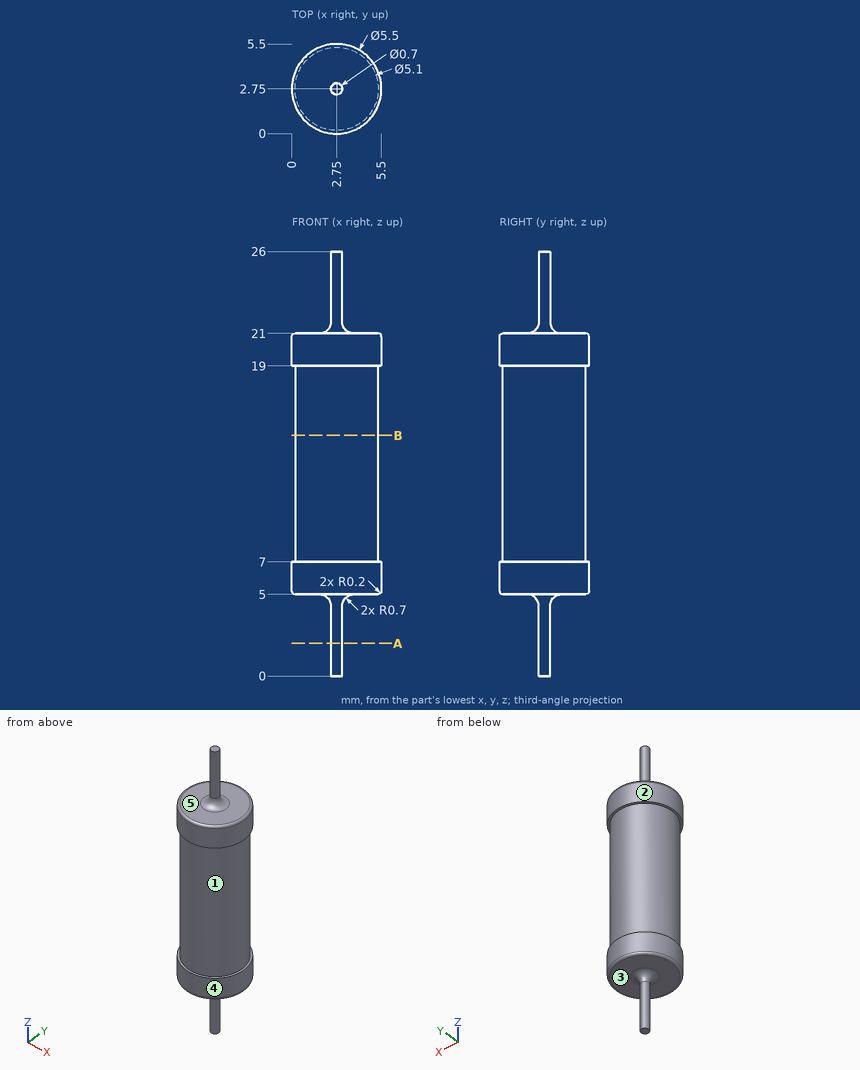
Design review of the part shown in the three views and the two pictorial views. Dimensions are in mm from the part's minimum x, y and z. A direction names the side the tool comes from. Coordinates: 2 decimals unless noted, no trailing zeros. Order: outer loops, then holes, each group sorted by start corner. A loop starts at its lowest first (then second) coordinate and runs counter-clockwise, first axis right, second up.
Item 1: For line 1 (Z direction, x = 4.5, y = 1.5); line 2 (Y direction, x = 2.75, z = 15); line 3 (Y direction, x = 0.45, z = 17), list the stretches that pass through material, from the lowest coordinate up.
Item 2: The part is to be moulded in two halves that separate along Z. For the marked faces 1, 2 and 3, say which applies: pulls with the +Z half, pulls with the -Z half, needs draft (parallel to the pull), parting line crosses it, or undercut.
Item 3: For the marked faces 4 and 5, list the 3-axis set-ups (+Z, -Z, +X, -X, +Y, -Y) from which the entire face can be reached by the end or side of a thin tool; tool diameter is ignored.
Item 4: Take a section at A-A, the plane z = 2. Write out the cut boundary in (x, y), then the cut area to 3 significant figures.
Item 5: For pin 1 Ø1 at (x, z) = (1.5, 11.5) entering from -Y; pin 2 Ø1.5 at (y, z) = (2, 7.5) entering from +X; pin 3 Ø1.5 at (x, y) = (4.5, 5) entering from -Z, all flat-tipped, find the tip position at first contact; note any pin that passes through.
Item 6: Take a section at B-B, the plane z = 14.75. Write out the cut boundary in (x, y).
The answers:
1. line 1: z = 5 to 21
1. line 2: y = 0.2 to 5.3
1. line 3: y = 1.65 to 3.85
2. face 1: undercut
2. face 2: needs draft
2. face 3: pulls with the -Z half
3. face 4: +Z, -Z
3. face 5: +Z
4. outline: circle Ø0.7 at (2.75, 2.75)
4. area: 0.385 mm2
5. pin 1: stops at y = 0.31
5. pin 2: stops at x = 5.49
5. pin 3: stops at z = 5
6. outline: circle Ø5.1 at (2.75, 2.75)
